```python
from build123d import *

# Parameters (mm, degrees)
SKETCH_2_R               = 5
EXTRUDE_1_DEPTH          = 10
PATTERN_CIRCULAR_1_COUNT = 6
EXTRUDE_2_DEPTH          = 7
SKETCH_4_R               = 1.4
CUT_EXTRUDE_1_DEPTH      = 53.086466711
PATTERN_CIRCULAR_2_COUNT = 6
SKETCH_5_R               = 5.5
EXTRUDE_3_DEPTH          = 5
SKETCH_7_R               = 7
CUT_EXTRUDE_3_DEPTH      = 1.5
CUT_EXTRUDE_3_DRAFT      = -40
SKETCH_8_R               = 1.5
CUT_EXTRUDE_4_DEPTH      = 53.93628259
SKETCH_10_R              = 1.25
CUT_EXTRUDE_6_DEPTH      = 54.366656391
PATTERN_CIRCULAR_3_COUNT = 6
SKETCH_11_R              = 2.5
CUT_EXTRUDE_7_DEPTH      = 54.366656391
PATTERN_CIRCULAR_4_COUNT = 2
CUT_EXTRUDE_8_DEPTH      = 8
PATTERN_CIRCULAR_5_COUNT = 6
CUT_EXTRUDE_9_DEPTH      = 8


with BuildPart() as part:
    # 草图1 → 旋转1 (revolve)
    with BuildSketch(Plane(origin=(0, 0, 0), x_dir=(1, 0, 0), z_dir=(0, 1, 0)), mode=Mode.PRIVATE) as revolve_1_sk:
        with BuildLine():
            Line((25, 10), (25, -10))
            Line((25, -10), (31, -10))
            ThreePointArc((31, -10), (35.787135539, -6.443375673), (33.763853992, -0.833333333))
            ThreePointArc((33.763853992, -0.833333333), (33.31662479, 0), (33.763853992, 0.833333333))
            ThreePointArc((33.763853992, 0.833333333), (35.787135539, 6.443375673), (31, 10))
            Line((31, 10), (25, 10))
        make_face()
    revolve(revolve_1_sk.sketch.rotate(Axis((0, 0, -146.934042126), (0, 0, 1)), 180), axis=Axis((0, 0, -146.934042126), (0, 0, 1)))

    # 草图2 → 凸台-拉伸1 (add)
    with BuildSketch(Plane.XY.offset(6)):
        with Locations((0, 21.5)):
            Circle(SKETCH_2_R)
    extrude_1 = extrude(amount=-EXTRUDE_1_DEPTH)

    # 阵列(圆周)1: 凸台-拉伸1 ×6 about axis
    pattern_circular_1_axis = Axis((0, 0, 0), (0, 0, 1))
    for i in range(1, PATTERN_CIRCULAR_1_COUNT):
        add(extrude_1.rotate(pattern_circular_1_axis, i * 360 / PATTERN_CIRCULAR_1_COUNT))

    # 草图3 → 凸台-拉伸2 (add)
    with BuildSketch(Plane.XY.offset(6)):
        with BuildLine():
            Line((-8.082903769, 0), (-10.874355653, -4.834936491))
            Line((-10.874355653, -4.834936491), (-15.051918724, -7.246853654))
            ThreePointArc((-15.051918724, -7.246853654), (-14.289419162, -8.25), (-13.801918724, -9.411917163))
            Line((-13.801918724, -9.411917163), (-9.624355653, -7))
            Line((-9.624355653, -7), (-4.041451884, -7))
            Line((-4.041451884, -7), (-1.25, -11.834936491))
            Line((-1.25, -11.834936491), (-1.25, -16.658770817))
            ThreePointArc((-1.25, -16.658770817), (0, -16.5), (1.25, -16.658770817))
            Line((1.25, -16.658770817), (1.25, -11.834936491))
            Line((1.25, -11.834936491), (4.041451884, -7))
            Line((4.041451884, -7), (9.624355653, -7))
            Line((9.624355653, -7), (13.801918724, -9.411917163))
            ThreePointArc((13.801918724, -9.411917163), (14.289419162, -8.25), (15.051918724, -7.246853654))
            Line((15.051918724, -7.246853654), (10.874355653, -4.834936491))
            Line((10.874355653, -4.834936491), (8.082903769, 0))
            Line((8.082903769, 0), (10.874355653, 4.834936491))
            Line((10.874355653, 4.834936491), (15.051918724, 7.246853654))
            ThreePointArc((15.051918724, 7.246853654), (14.289419162, 8.25), (13.801918724, 9.411917163))
            Line((13.801918724, 9.411917163), (9.624355653, 7))
            Line((9.624355653, 7), (4.041451884, 7))
            Line((4.041451884, 7), (1.25, 11.834936491))
            Line((1.25, 11.834936491), (1.25, 16.658770817))
            ThreePointArc((1.25, 16.658770817), (0, 16.5), (-1.25, 16.658770817))
            Line((-1.25, 16.658770817), (-1.25, 11.834936491))
            Line((-1.25, 11.834936491), (-4.041451884, 7))
            Line((-4.041451884, 7), (-9.624355653, 7))
            Line((-9.624355653, 7), (-13.801918724, 9.411917163))
            ThreePointArc((-13.801918724, 9.411917163), (-14.289419162, 8.25), (-15.051918724, 7.246853654))
            Line((-15.051918724, 7.246853654), (-10.874355653, 4.834936491))
            Line((-10.874355653, 4.834936491), (-8.082903769, 0))
        make_face()
    extrude(amount=-EXTRUDE_2_DEPTH)

    # 草图4 → 切除-拉伸1 (cut, through all)
    with BuildSketch(Plane(origin=(0, 0, -1), x_dir=(-1, 0, 0), z_dir=(0, 0, -1))):
        with Locations((0, 8.5)):
            Circle(SKETCH_4_R)
    cut_extrude_1 = extrude(amount=-CUT_EXTRUDE_1_DEPTH, mode=Mode.SUBTRACT)

    # 阵列(圆周)2: 切除-拉伸1 ×6 about axis
    pattern_circular_2_axis = Axis((0, 0, 0), (0, 0, 1))
    for i in range(1, PATTERN_CIRCULAR_2_COUNT):
        add(cut_extrude_1.rotate(pattern_circular_2_axis, i * 360 / PATTERN_CIRCULAR_2_COUNT), mode=Mode.SUBTRACT)

    # 草图5 → 凸台-拉伸3 (add)
    with BuildSketch(Plane(origin=(0, 0, -1), x_dir=(-1, 0, 0), z_dir=(0, 0, -1))):
        with Locations(Location((0, 0, 0), (0, 0, 180))):
            Circle(SKETCH_5_R)
    extrude(amount=EXTRUDE_3_DEPTH)


with BuildPart() as cut_extrude_3_tool:
    # 草图7 → 切除-拉伸3 (with draft: the straight prism first)
    with BuildSketch(Plane.XY.offset(6)):
        Circle(SKETCH_7_R)
    extrude(amount=-CUT_EXTRUDE_3_DEPTH)
    # 切除-拉伸3: the draft: its side faces are tilted about the plane it starts from
    cut_extrude_3_sides = [cut_extrude_3_tool.faces().sort_by_distance(p)[0] for p in [
        (-7, 0, 5.25),
    ]]
    draft(cut_extrude_3_sides, Plane.XY.offset(6), CUT_EXTRUDE_3_DRAFT)


with BuildPart() as part_1:
    add(part.part)

    # 切除-拉伸3: cut by cut_extrude_3_tool
    add(cut_extrude_3_tool.part, mode=Mode.SUBTRACT)

    # 草图8 → 切除-拉伸4 (cut, through all)
    with BuildSketch(Plane.XY.offset(4.5)):
        Circle(SKETCH_8_R)
    extrude(amount=-CUT_EXTRUDE_4_DEPTH, mode=Mode.SUBTRACT)

    # 草图10 → 切除-拉伸6 (cut, through all)
    with BuildSketch(Plane.XY.offset(6)):
        with Locations((0, 21.5)):
            Circle(SKETCH_10_R)
    cut_extrude_6 = extrude(amount=-CUT_EXTRUDE_6_DEPTH, mode=Mode.SUBTRACT)

    # 阵列(圆周)3: 切除-拉伸6 ×6 about axis
    pattern_circular_3_axis = Axis((0, 0, 0), (0, 0, 1))
    for i in range(1, PATTERN_CIRCULAR_3_COUNT):
        add(cut_extrude_6.rotate(pattern_circular_3_axis, i * 360 / PATTERN_CIRCULAR_3_COUNT), mode=Mode.SUBTRACT)

    # 草图11 → 切除-拉伸7 (cut, through all)
    with BuildSketch(Plane.XY.offset(6)):
        with Locations((0, 21.5)):
            Circle(SKETCH_11_R)
    cut_extrude_7 = extrude(amount=-CUT_EXTRUDE_7_DEPTH, mode=Mode.SUBTRACT)

    # 阵列(圆周)4: 切除-拉伸7 ×2 about axis
    pattern_circular_4_axis = Axis((0, 0, 0), (0, 0, 1))
    for i in range(1, PATTERN_CIRCULAR_4_COUNT):
        add(cut_extrude_7.rotate(pattern_circular_4_axis, i * 360 / PATTERN_CIRCULAR_4_COUNT), mode=Mode.SUBTRACT)

    # 草图12 → 切除-拉伸8 (cut)
    with BuildSketch(Plane.XY.offset(6)):
        Polygon((20.062921854, 8.25), (21.506297527, 10.75), (20.062921854, 13.25), (17.176170508, 13.25), (15.732794835, 10.75), (17.176170508, 8.25), align=None)
    cut_extrude_8 = extrude(amount=-CUT_EXTRUDE_8_DEPTH, mode=Mode.SUBTRACT)

    # 阵列(圆周)5: 切除-拉伸8 ×6 about axis, 2 skipped
    pattern_circular_5_axis = Axis((0, 0, 0), (0, 0, -1))
    add([cut_extrude_8.rotate(pattern_circular_5_axis, i * 360 / PATTERN_CIRCULAR_5_COUNT) for i in range(1, PATTERN_CIRCULAR_5_COUNT) if i not in (2, 5)], mode=Mode.SUBTRACT)

    # 草图9 → 切除-拉伸9 (cut)
    with BuildSketch(Plane(origin=(0, 0, -6), x_dir=(-1, 0, 0), z_dir=(0, 0, -1))):
        Polygon((3.5, 0), (1.75, 3.031088913), (-1.75, 3.031088913), (-3.5, 0), (-1.75, -3.031088913), (1.75, -3.031088913), align=None)
    extrude(amount=-CUT_EXTRUDE_9_DEPTH, mode=Mode.SUBTRACT)


solid = part_1.part
```
Work out the finished part from the listing and answer in its coordinate system (mm). A direction names the side the tool comes from. Give positions to 0.01 mm unless a question says otherwise; leave off trailing zeros. Write each loop counter-clockwise with the first axis right and the second up, starting at its lowest first coordinate (ties: lowest second). Pieces come first, ordered by that corner, then holes. Notation, with made-up numbers: (67, -13) - (81, -13) arc R22 ccw to (81, 20) - close; hole circle Ø9 at (76, 35). An arc over 180 degrees is marked (long way). Use one line per item in the form item = value.
1. Each of these flat-tipped pins is pushed along its axis until it touches: pin 1 Ø1.8 at (x, y) = (0, 1.5) entering from -Z; pin 2 Ø4 at (x, y) = (-18.62, -10.75) entering from +Z; pin 3 Ø1.4 at (x, z) = (-18.5, 2.5) entering from +Y. Where does it stop, or does it pass through?
Filled in:
pin_1 = 2
pin_2 = -2
pin_3 = 30.69
2. A cutting plane is placed at B-B (z = -8). Write down the section's boundary in (x, y).
Filled in:
outline = circle Ø70 at (0, 0); hole circle Ø50 at (0, 0)
3. Determine the mould class of faces 4 (the face through (-2, 0, 2)), 5 (the face through (-1.19, 5.37, -3.46)) for opening direction X: released by +X, released by -X, zero draft, split by the parting line, or undercut.
Filled in:
face_4 = undercut
face_5 = undercut
4. For faces 1 (the face through (19, -9, -4)), 2 (the face through (-20.775, 12.017, 2.056)), 3 (the face through (2.6, -9.5, 2.5)), determine the directions among +Z, -Z, +X, -X, +Y, -Y from which every point of the face is accessible in a straight line to the end or side of a thin tool.
Filled in:
face_1 = -Z
face_2 = +Z
face_3 = +Z, -Z
5. A cutting plane is placed at A-A (x = 0). State how many separate pieces and enclosed holes the cut face has, and give its area (3 significant figures).
Filled in:
separate_pieces = 6
enclosed_holes = 0
area = 641 mm^2
6. Consider L1, parallel to Y at x = -18, z = -1.5; L2, parallel to X at y = -13.5, z = 1.75; L3, parallel to X at y = -2, z = -5. Determine where each line is inside the solid, lowest interval first.
Filled in:
L1 = -29.51 to -17.35, -15.71 to -13.25, -8.25 to -5.79, 5.79 to 8.25, 13.25 to 15.71, 17.35 to 29.51
L2 = -32.07 to -14.44, -1.25 to 1.25, 14.44 to 32.07
L3 = -35.94 to -24.92, -5.12 to -2.35, 2.35 to 5.12, 24.92 to 35.94
